```python
from build123d import *

# Parameters (mm, degrees)
F0_R     = 3
F0_R_2   = 21.5
F0_R_3   = 12.5
F1_DEPTH = 12
F2_SIZE  = 10
F3_R     = 5.25
F3_R_2   = 3
F4_DEPTH = 6


with BuildPart() as f1:
    # F0 (on Front) → F1 (new body)
    with BuildSketch(Plane.XZ):
        Polygon((0, 145), (0, 0), (80, 0), (80, 220), (-55, 220), (-55, 145), align=None)
        with Locations((6, 20)):
            Circle(F0_R, mode=Mode.SUBTRACT)
        with Locations((6, 80)):
            Circle(F0_R, mode=Mode.SUBTRACT)
        with Locations((74, 20)):
            Circle(F0_R, mode=Mode.SUBTRACT)
        with Locations((74, 80)):
            Circle(F0_R, mode=Mode.SUBTRACT)
        with Locations((-32.5, 182.5)):
            Circle(F0_R_2, mode=Mode.SUBTRACT)
        with Locations((15.751263, 157.751263)):
            Circle(F0_R, mode=Mode.SUBTRACT)
        with Locations((65.248737, 157.751263)):
            Circle(F0_R, mode=Mode.SUBTRACT)
        with Locations((40.5, 182.5)):
            Circle(F0_R_3, mode=Mode.SUBTRACT)
        with Locations((15.751263, 207.248737)):
            Circle(F0_R, mode=Mode.SUBTRACT)
        with Locations((65.248737, 207.248737)):
            Circle(F0_R, mode=Mode.SUBTRACT)
    extrude(amount=F1_DEPTH)

    # F2
    f2_edges = [f1.edges().sort_by_distance(p)[0] for p in [
        (-55, -6, 220),
        (-55, -6, 145),
    ]]
    chamfer(f2_edges, length=F2_SIZE)

    # F3 (on face) → F4 (cut)
    with BuildSketch(Plane.XZ.offset(12)):
        with Locations((6, 80)):
            Circle(F3_R)
        with Locations((6, 80)):
            Circle(F3_R_2, mode=Mode.SUBTRACT)
        with Locations((74, 80)):
            Circle(F3_R)
        with Locations((74, 80)):
            Circle(F3_R_2, mode=Mode.SUBTRACT)
        with Locations((74, 20)):
            Circle(F3_R)
        with Locations((74, 20)):
            Circle(F3_R_2, mode=Mode.SUBTRACT)
        with Locations((6, 20)):
            Circle(F3_R)
        with Locations((6, 20)):
            Circle(F3_R_2, mode=Mode.SUBTRACT)
    extrude(amount=-F4_DEPTH, mode=Mode.SUBTRACT)


solid = f1.part
```
Could you check a few things on this model? Use its own coordinates, in mm. A direction names the side the tool comes from. Give positions to 0.01 mm unless a question says otherwise; leave off trailing zeros. Loops run counter-clockwise (first coordinate to the right, second up) from the corner with the lowest first, then second, coordinate; pieces in that order, holes last. Notation, with made-up numbers: (-24, 52.5) - (23, 52.5) arc R27 ccw to (23, 83.5) - close; hole circle Ø11 at (-12, -6). An arc over 180 degrees is marked (long way). Use one line per item in the form item = value.
1. Thinking about a two-plate mould opening in X: for faces 4 (the face through (18, -6, 220)), 5 (the face through (80, -6, 108)), 6 (the face through (63.04, -5.92, 209.28)), 7 (the face through (-50, -6, 215)), which applies, released by +X, released by -X, zero draft, split by the parting line, or undercut?
Response values:
face_4 = zero draft
face_5 = released by +X
face_6 = undercut
face_7 = released by -X
2. I want a section at C-C (x = -32.5). Please give me the cut outline in (y, z).
Response values:
outline = (-12, 145) - (0, 145) - (0, 161) - (-12, 161) - close; (-12, 204) - (0, 204) - (0, 220) - (-12, 220) - close
3. I need wall thicknesses on probe 1 along Z at (x, y) = (65.5, -5.25); probe 2 along Z at (x, y) = (74, -7.25); probe 3 along X at (y, z) = (-10.75, 173). Which ranges of each line are inside material? Lowest first, please.
Response values:
probe_1 = 0 to 154.76, 160.74 to 204.26, 210.24 to 220
probe_2 = 0 to 14.75, 25.25 to 74.75, 85.25 to 220
probe_3 = -55 to -51.79, -13.21 to 32.38, 48.62 to 80
4. I want a section at D-D (y = -2.75). Give the number of separate pieces and of enclosed holes in the cut face, and give its area (3 significant figures).
Response values:
separate_pieces = 1
enclosed_holes = 10
area = 19,500 mm²
5. I'm going to push flat-ended pins straight in: pin 1 Ø3 at (x, z) = (6, 20.5) entering from -Y; pin 2 Ø6.5 at (x, z) = (6, 80) entering from -Y; pin 3 Ø6 at (y, z) = (-3.5, 57) entering from -X; pin 4 Ø3.5 at (x, y) = (-22.5, -7) entering from -Z. Where does each tip first touch, or does it pass through?
Response values:
pin_1 = through
pin_2 = -6
pin_3 = 0
pin_4 = 145
6. I want a section at A-A (z = 20). Please give me the cut outline in (x, y).
Response values:
outline = (0, -12) - (0.75, -12) - (0.75, -6) - (3, -6) - (3, 0) - (0, 0) - close; (9, -6) - (11.25, -6) - (11.25, -12) - (68.75, -12) - (68.75, -6) - (71, -6) - (71, 0) - (9, 0) - close; (77, -6) - (79.25, -6) - (79.25, -12) - (80, -12) - (80, 0) - (77, 0) - close
7. I want a section at B-B (x = 6). Please give me the cut outline in (y, z).
Response values:
outline = (-12, 0) - (0, 0) - (0, 17) - (-6, 17) - (-6, 14.75) - (-12, 14.75) - close; (-12, 25.25) - (-6, 25.25) - (-6, 23) - (0, 23) - (0, 77) - (-6, 77) - (-6, 74.75) - (-12, 74.75) - close; (-12, 85.25) - (-6, 85.25) - (-6, 83) - (0, 83) - (0, 220) - (-12, 220) - close
8. On a 3-axis mill with a long thin cutter (end or side, diameter ignored), from which of +Z, -Z, +X, -X, +Y, -Y can I reach the whole of each face in a straight line? I mean faces 1 (the face through (15.361, -5.916, 210.223)), 2 (the face through (68.755, -9.042, 80.231)), 3 (the face through (-23, -6, 145)). Say none if no direction works.
Response values:
face_1 = +Y, -Y
face_2 = -Y
face_3 = -Z, -X, +Y, -Y
